Part print with two shaded views. Sizes in mm from the minimum x, y, z corner. Round coordinates to 2 decimals unless told otherwise and drop trailing zeros. Write each loop counter-clockwise with the first axis right and the second up, starting at its lowest first coordinate (ties: lowest second). Pieces come first, ordered by that corner, then holes. Notation, with made-up numbers: (39.5, 42) -> (50.5, 42) arc R28 cw to (50.5, 65) -> close; hole circle Ø6 at (8.5, 21). An arc over 180 degrees is marked (long way). Put each result on its own line as item: value. Start each with the question number.
1. Drill centre lines: line 1 (Z direction, x = 16.25, y = 170); line 2 (Y direction, x = 13, z = 45); line 3 (Y direction, x = 14.25, z = 70). Where is each one in solid material? Low to high. Write a range as from..to.
2. Saw through at C-C on z = 75. List the corners of the cut face in (x, y), and give its area (3 significant figures).
3. Saw through at B-B on y = 170. List the corners of the cut face in (x, z).
4. Pull direction Y, two halves, no side cores. Call the marked faces 1 and 2: pulls with the +Y half, pulls with the -Y half, needs draft (parallel to the pull), parting line crosses it, or undercut.
5. Saw through at A-A on x = 14.75. List the corners of the cut face in (y, z).
6. Flat gauge pin, fed straight in: P1, Ø4, axis at y = 170, z = 105, coming from the +X side. Where does the tip first touch, or does it go through?
7. Saw through at D-D on z = 35. List the corners of the cut face in (x, y), and give its area (3 significant figures).
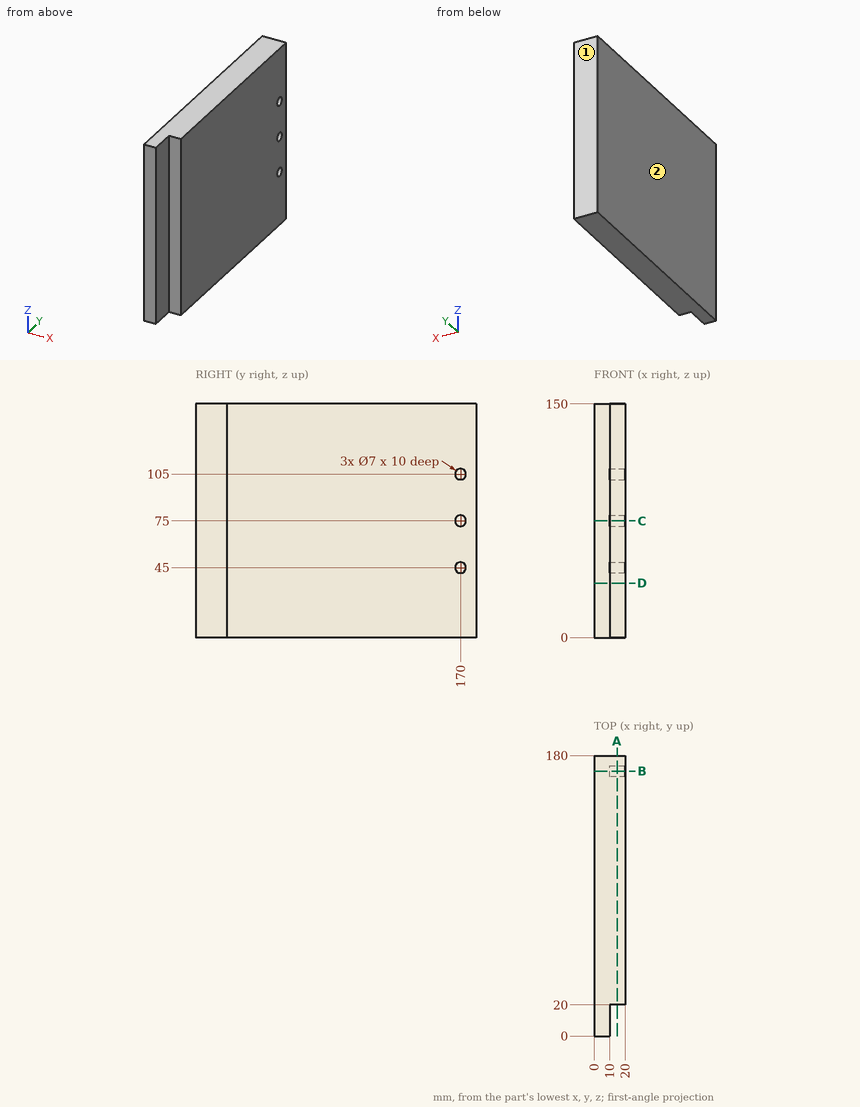
Return value:
1. line 1: z = 0..41.5, 48.5..71.5, 78.5..101.5, 108.5..150
1. line 2: y = 20..166.5, 173.5..180
1. line 3: y = 20..180
2. outline: (0, 0) -> (10, 0) -> (10, 20) -> (20, 20) -> (20, 166.5) -> (10, 166.5) -> (10, 173.5) -> (20, 173.5) -> (20, 180) -> (0, 180) -> close
2. area: 3,330 mm^2
3. outline: (0, 0) -> (20, 0) -> (20, 41.5) -> (10, 41.5) -> (10, 48.5) -> (20, 48.5) -> (20, 71.5) -> (10, 71.5) -> (10, 78.5) -> (20, 78.5) -> (20, 101.5) -> (10, 101.5) -> (10, 108.5) -> (20, 108.5) -> (20, 150) -> (0, 150) -> close
4. face 1: pulls with the +Y half
4. face 2: needs draft
5. outline: (20, 0) -> (180, 0) -> (180, 150) -> (20, 150) -> close; hole circle Ø7 at (170, 45); hole circle Ø7 at (170, 75); hole circle Ø7 at (170, 105)
6. P1: stops at x = 10
7. outline: (0, 0) -> (10, 0) -> (10, 20) -> (20, 20) -> (20, 180) -> (0, 180) -> close
7. area: 3,400 mm^2
